Part model, mm, in its own coordinate system. Face numbers are marked on the shaded views. Coordinates: 2 decimals unless noted, no trailing zeros. Loops run counter-clockwise (first coordinate to the right, second up) from the corner with the lowest first, then second, coordinate; pieces in that order, holes last. Notation, with made-up numbers: (38.25, 14.5) - (61.25, 14.5) arc R16 ccw to (61.25, 20.5) - close; hole circle Ø4 at (5.25, -21.75). An arc over 180 degrees is marked (long way). Use a Markdown table: item, result. Add a question column.
1) Drop flat-ended pins along their axis: P1, Ø3, axis at x = 527, z = 4.5, coming from the -Y side; P2, Ø1.5, axis at x = 236, y = 13, coming from the -Z side; P3, Ø3, axis at x = 600, y = -2.5, coming from the +Z side. Give the stop position or say it passes through.
2) Pull direction Z, two halves, no side cores. Call the marked faces 1 and 2: +Z half, -Z half, draft (parallel to the pull), parting line (faces both ways), or undercut.
3) Band-saw the part on A-A (z = 0). Give the cut face in (x, y), plus the area to 3 significant figures.
4) Probe probe 1 along Y at (x, z) = (5, 0); probe 2 along Y at (x, z) = (396, 0); probe 3 along Z at (x, y) = (102, -14). List the from-to ranges inside material, lowest first. Write a range as [from, to].
5) Band-saw the part on C-C (x = 691.5). Give the cut face in (y, z).
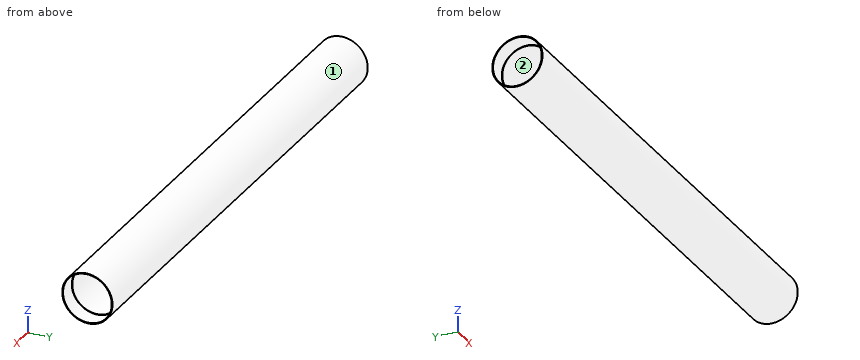
from build123d import *

# Parameters (mm, degrees)
SKETCH1_R           = 37.6555
BOSS_EXTRUDE1_DEPTH = 742.3404
SKETCH4_R           = 36.5
CUT_EXTRUDE2_DEPTH  = 25.4
CUT_EXTRUDE3_START  = -25.4
SKETCH5_R           = 36.5
CUT_EXTRUDE3_DEPTH  = 25.4
SKETCH6_R           = 35.75
CUT_EXTRUDE4_DEPTH  = 719.915440447


with BuildPart() as part:
    # Sketch1 → Boss-Extrude1 (new body)
    with BuildSketch(Plane(origin=(0, 0, 0), x_dir=(0, 0, -1), z_dir=(1, 0, 0))):
        Circle(SKETCH1_R)
    extrude(amount=BOSS_EXTRUDE1_DEPTH)

    # Sketch4 → Cut-Extrude2 (cut)
    with BuildSketch(Plane(origin=(742.3404, 0, 0), x_dir=(0, 0, -1), z_dir=(1, 0, 0))):
        Circle(SKETCH4_R)
    extrude(amount=-CUT_EXTRUDE2_DEPTH, mode=Mode.SUBTRACT)

    # Sketch5 → Cut-Extrude3 (cut)
    with BuildSketch(Plane.ZY.offset(CUT_EXTRUDE3_START)):
        with Locations(Location((0, 0, 0), (0, 0, 180))):
            Circle(SKETCH5_R)
    extrude(amount=CUT_EXTRUDE3_DEPTH, mode=Mode.SUBTRACT)

    # Sketch6 → Cut-Extrude4 (cut, through all)
    with BuildSketch(Plane(origin=(716.9404, 0, 0), x_dir=(0, 0, -1), z_dir=(1, 0, 0))):
        Circle(SKETCH6_R)
    extrude(amount=-CUT_EXTRUDE4_DEPTH, mode=Mode.SUBTRACT)


solid = part.part
Answer block:
| question | item | result |
|---|---|---|
| 1 | P1 | y = -37.54 |
| 1 | P2 | z = -35.61 |
| 1 | P3 | z = 37.64 |
| 2 | face 1 | parting line |
| 2 | face 2 | undercut |
| 3 | outline | (0, -37.66) - (742.34, -37.66) - (742.34, -36.5) - (716.94, -36.5) - (716.94, -35.75) - (25.4, -35.75) - (25.4, -36.5) - (0, -36.5) - close; (0, 36.5) - (25.4, 36.5) - (25.4, 35.75) - (716.94, 35.75) - (716.94, 36.5) - (742.34, 36.5) - (742.34, 37.66) - (0, 37.66) - close |
| 3 | area | 2,750 mm2 |
| 4 | probe 1 | [-37.66, -36.5], [36.5, 37.66] |
| 4 | probe 2 | [-37.66, -35.75], [35.75, 37.66] |
| 4 | probe 3 | [-34.96, -32.89], [32.89, 34.96] |
| 5 | outline | circle Ø75.31 at (0, 0); hole circle Ø71.5 at (0, 0) |
